Geometry: final body of the model. Coordinates: model frame, mm. Face numbers are marked on the shaded views. A direction names the side the tool comes from. Round coordinates to 2 decimals unless told otherwise and drop trailing zeros. Loops run counter-clockwise (first coordinate to the right, second up) from the corner with the lowest first, then second, coordinate; pieces in that order, holes last. Notation, with made-up numbers: (-23, -26) -> (14, -26) arc R9 cw to (14, -13) -> close; hole circle Ø10 at (-8, 51.25). An arc over 180 degrees is marked (long way). Answer in a Markdown table with one row per item.
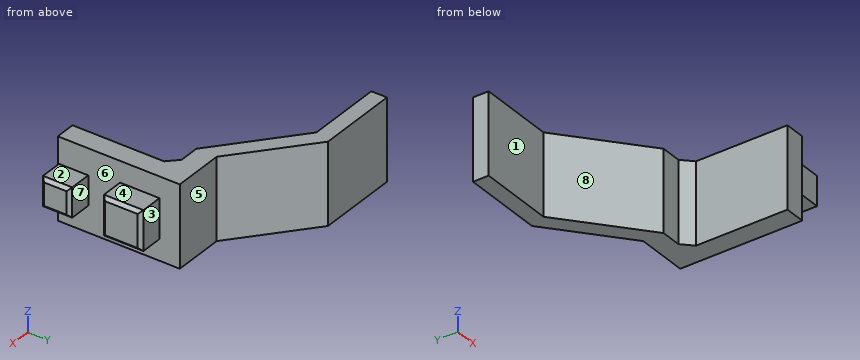
```python
from build123d import *

# Parameters (mm, degrees)
BOSS_EXTRUDE1_DEPTH = 4
SKETCH1_3_W         = 2.5
SKETCH1_3_H         = 3.875
BOSS_EXTRUDE2_DEPTH = 1.9375
SKETCH1_4_W         = 2.5
SKETCH1_4_H         = 2.875
BOSS_EXTRUDE3_DEPTH = 1.4375
CHAMFER1_SIZE       = 0.325


with BuildPart() as part:
    # Sketch1 → Boss-Extrude1 (new, symmetric)
    with BuildSketch(Plane.XY):
        Polygon((-5, 10), (-3, 10), (-2, 9), (-2, 0), (0, 0), (0, 12), (-5, 12), align=None)
        Polygon((-20, 16.335837533), (-12.550757142, 16.335837533), (-5, 10), (-5, 12), (-12, 17.873697418), (-20, 17.873697418), align=None)
    extrude(amount=BOSS_EXTRUDE1_DEPTH, both=True)

    # Sketch1_3 → Boss-Extrude2 (add, symmetric)
    with BuildSketch(Plane.XY):
        with Locations((1.25, 8.0625)):
            Rectangle(SKETCH1_3_W, SKETCH1_3_H)
    extrude(amount=BOSS_EXTRUDE2_DEPTH, both=True)

    # Sketch1_4 → Boss-Extrude3 (add, symmetric)
    with BuildSketch(Plane.XY):
        with Locations((1.25, 1.5625)):
            Rectangle(SKETCH1_4_W, SKETCH1_4_H)
    extrude(amount=BOSS_EXTRUDE3_DEPTH, both=True)

    # Chamfer1
    chamfer1_edges = [part.edges().sort_by_distance(p)[0] for p in [
        (2.5, 8.0625, 1.9375),
        (2.5, 6.125, 0),
        (2.5, 10, 0),
        (2.5, 8.0625, -1.9375),
        (2.5, 1.5625, 1.4375),
        (2.5, 0.125, 0),
        (2.5, 3, 0),
        (2.5, 1.5625, -1.4375),
    ]]
    chamfer(chamfer1_edges, length=CHAMFER1_SIZE)


solid = part.part
```
Item 1: Cut plane C-C (x = -0.75). Output: boundary loops of the cut face in (y, z).
Answer:
| item | result |
|---|---|
| outline | (0, -4) -> (12, -4) -> (12, 4) -> (0, 4) -> close |
Item 2: Cut plane B-B (y = 2). Output: boundary loops of the cut face in (x, z) (1 decimal), then the cut area to 3 significant figures.
Answer:
| item | result |
|---|---|
| outline | (-2, -4) -> (0, -4) -> (0, -1.4) -> (2.2, -1.4) -> (2.5, -1.1) -> (2.5, 1.1) -> (2.2, 1.4) -> (0, 1.4) -> (0, 4) -> (-2, 4) -> close |
| area | 23.1 mm² |
Item 3: Cut plane A-A (z = 0.5). Output: boundary loops of the cut face in (x, y) (3 decimals), then the cut area to 3 significant figures.
Answer:
| item | result |
|---|---|
| outline | (-20, 16.336) -> (-12.551, 16.336) -> (-5, 10) -> (-3, 10) -> (-2, 9) -> (-2, 0) -> (0, 0) -> (0, 0.125) -> (2.175, 0.125) -> (2.5, 0.45) -> (2.5, 2.675) -> (2.175, 3) -> (0, 3) -> (0, 6.125) -> (2.175, 6.125) -> (2.5, 6.45) -> (2.5, 9.675) -> (2.175, 10) -> (0, 10) -> (0, 12) -> (-5, 12) -> (-12, 17.874) -> (-20, 17.874) -> close |
| area | 73.6 mm² |
Item 4: Pin query (flat end, axial travel): pin 1 Ø1.7 at (x, y) = (1, 7.5) entering from -Z; pin 2 Ø2 at (x, z) = (-15.5, 0) entering from -Y; pin 3 Ø1.1 at (x, y) = (1.5, 2.5) entering from -Z. Return the tip coordinate at first contact, or that it passes through.
Answer:
| item | result |
|---|---|
| pin 1 | stops at z = -1.94 |
| pin 2 | stops at y = 16.34 |
| pin 3 | stops at z = -1.44 |
Item 5: Cut plane D-D (z = 3.25). Output: boundary loops of the cut face in (x, y), then the cut area to 3 significant figures.
Answer:
| item | result |
|---|---|
| outline | (-20, 16.34) -> (-12.55, 16.34) -> (-5, 10) -> (-3, 10) -> (-2, 9) -> (-2, 0) -> (0, 0) -> (0, 12) -> (-5, 12) -> (-12, 17.87) -> (-20, 17.87) -> close |
| area | 56.9 mm² |
Item 6: Line query: probe 1 along Z at (x, y) = (0.75, 1); probe 2 along Y at (x, z) = (-18, -3); probe 3 along X at (y, z) = (1, 3.75). Output: solid intervals per line, ascending. Write a range as [from, to].
Answer:
| item | result |
|---|---|
| probe 1 | z = [-1.44, 1.44] |
| probe 2 | y = [16.34, 17.87] |
| probe 3 | x = [-2, 0] |
Item 7: Reachability of the marked faces 1, 2, 3 and 4 from +Z, -Z, +X, -X, +Y, -Y: full face, straight path, thin tool, end or side. Return the list, or none.
Answer:
| item | result |
|---|---|
| face 1 | +Z, -Z, -X, -Y |
| face 2 | +Z, +X, -Y |
| face 3 | +Z, -Z, +X, +Y |
| face 4 | +Z, +X, +Y, -Y |
Item 8: Draft query along Y for the marked faces 5, 6, 7 and 8. Return one class per face: pulls with the +Y half, pulls with the -Y half, needs draft (parallel to the pull), parting line crosses it, or undercut.
Answer:
| item | result |
|---|---|
| face 5 | pulls with the +Y half |
| face 6 | undercut |
| face 7 | undercut |
| face 8 | pulls with the -Y half |
